```python
from build123d import *

# Parameters (mm, degrees)
BOSS_EXTRUDE3_DEPTH = 9
SKETCH5_R           = 5.25
CUT_EXTRUDE4_DEPTH  = 18
SKETCH6_R           = 5.25
CUT_EXTRUDE5_DEPTH  = 18
FILLET1_R           = 5


with BuildPart() as part:
    # Sketch1 → Boss-Extrude3 (new, symmetric)
    with BuildSketch(Plane.XY):
        with BuildLine():
            Line((-24.520010838, 91.781093197), (-20.91393225, 82.386937301))
            ThreePointArc((-20.91393225, 82.386937301), (-70.050726033, 48.144530139), (-84.409715081, -10))
            Line((-84.409715081, -10), (-94.472218138, -10))
            ThreePointArc((-94.472218138, -10), (-78.291987919, 53.808592508), (-24.520010838, 91.781093197))
        make_face()
    extrude(amount=BOSS_EXTRUDE3_DEPTH, both=True)

    # Sketch5 → Cut-Extrude4 (cut)
    with BuildSketch(Plane(origin=(-34.044955207, 88.690140517, 0), x_dir=(0.9335804264972001, 0.35836794954530493, 0), z_dir=(-0.35836794954530493, 0.9335804264972001, 0))):
        with Locations(Location((0, 0, 0), (0, 0, 180))):
            Circle(SKETCH5_R)
    extrude(amount=-CUT_EXTRUDE4_DEPTH, mode=Mode.SUBTRACT)

    # Sketch6 → Cut-Extrude5 (cut)
    with BuildSketch(Plane.ZY.offset(95)):
        Circle(SKETCH6_R)
    extrude(amount=-CUT_EXTRUDE5_DEPTH, mode=Mode.SUBTRACT)

    # Fillet1
    fillet1_edges = [part.edges().sort_by_distance(p)[0] for p in [
        (-89.44096661, -10, 9),
        (-89.44096661, -10, -9),
        (-22.716971544, 87.084015249, -9),
        (-22.716971544, 87.084015249, 9),
    ]]
    fillet(fillet1_edges, radius=FILLET1_R)


solid = part.part
```
The listing builds one solid part. Answer for the finished solid, in the listing's coordinates (mm). Coordinates: 2 decimals unless noted, no trailing zeros. Write each loop counter-clockwise with the first axis right and the second up, starting at its lowest first coordinate (ties: lowest second). Pieces come first, ordered by that corner, then holes.
Q1. Section B-B, the plane z = 0 is taken. Write down the section's boundary in (x, y), then the cut area to 3 significant figures.
Returned:
outline: (-94.85, -5.25) arc R95 ccw to (-94.47, -10) - (-84.41, -10) arc R85 cw to (-84.84, -5.25) - close; (-94.85, 5.25) - (-84.84, 5.25) arc R85 cw to (-35.3, 77.32) - (-38.89, 86.67) arc R95 ccw to start; (-29.09, 90.44) - (-25.5, 81.08) arc R85 cw to (-20.91, 82.39) - (-24.52, 91.78) arc R95 ccw to start
area: 1,070 mm2
Q2. Find the intervals of material crossed by line 1 along Z through (x, y) = (-31, 82); line 2 along X through (y, z) = (84, -1); line 3 along X through (y, z) = (-2, 7.5), in increasing order.
Returned:
line 1: z = -9 to -5.23, 5.23 to 9
line 2: x = -44.37 to -37.77, -26.72 to -21.53
line 3: x = -94.98 to -84.98
Q3. Section A-A, the plane y = 0 is taken. Write down the section's boundary in (x, z), then the cut area to 3 significant figures.
Returned:
outline: (-95, -9) - (-85, -9) - (-85, -5.25) - (-95, -5.25) - close; (-95, 5.25) - (-85, 5.25) - (-85, 9) - (-95, 9) - close
area: 75.0 mm2
Q4. Given P1, Ø2, axis at y = 34.5, z = 3.5, coming from the -X side; P2, Ø8, axis at y = 47.5, z = 6.5, coming from the +X side; P3, Ø4, axis at y = 64, z = 4.5, coming from the -X side, each flat-ended and moving along its own axis, determine where each tip first touches the part or whether it passes through.
Returned:
P1: stops at x = -88.9
P2: stops at x = -67.62
P3: stops at x = -71.98
Q5. The mould has two halves that part along Z. Classify faces 1 (the flat face through (-70, 50, 9)), 2 (the cylindrical face through (-90, 1.6, 5)), 3 (the cylindrical face through (-24.1, 86.7, -7.5)): released by +Z, released by -Z, zero draft, split by the parting line, or undercut.
Returned:
face 1: released by +Z
face 2: undercut
face 3: released by -Z
Q6. Section C-C, the plane x = -51 is taken. Write down the section's boundary in (y, z).
Returned:
outline: (68, -9) - (80.15, -9) - (80.15, 9) - (68, 9) - close
Q7. Section D-D, the plane y = 30 is taken. Write down the section's boundary in (x, z), then the cut area to 3 significant figures.
Returned:
outline: (-90.14, -9) - (-79.53, -9) - (-79.53, 9) - (-90.14, 9) - close
area: 191 mm2
